Solid Edge part; units mm, degrees
sketch "Sketch1" plane through (0, 0, 0) normal (0, -1, 0) x (1, 0, 0)
  line L0 (0, 50.8) -> (0, 0)
  line L1 (0, 0) -> (50.8, 0)
  line L2 (50.8, 0) -> (50.8, 1.905)
  arc A0 (50.8, 1.905) -> (47.9425, 4.7625) centre (47.9425, 1.905) ccw
  line L3 (47.9425, 4.7625) -> (10.4775, 4.7625)
  arc A1 (10.4775, 4.7625) -> (4.7625, 10.4775) centre (10.4775, 10.4775) cw
  line L4 (4.7625, 10.4775) -> (4.7625, 47.9425)
  arc A2 (4.7625, 47.9425) -> (1.905, 50.8) centre (1.905, 47.9425) ccw
  line L5 (1.905, 50.8) -> (0, 50.8)
extrude "Protrusion1" add sketch "Sketch1" against normal blind 34.925
The listing builds one solid part. Answer for the finished solid, in the listing's coordinates (mm). A direction names the side the tool comes from. Coordinates: 2 decimals unless noted, no trailing zeros. Order: outer loops, then holes, each group sorted by start corner. A loop starts at its lowest first (then second) coordinate and runs counter-clockwise, first axis right, second up. Notation, with made-up numbers: (62, 26.25) -> (98, 26.25) arc R10 ccw to (98, 39.25) -> close; hole circle Ø2 at (29, 10). An arc over 180 degrees is marked (long way). Answer in a Markdown table with one row per item. Add a question column.
Item 1: Find section C-C (x = 27.5). Write down the section's boundary in (y, z) (1 decimal), then the cut area to 3 significant figures.
Item 2: Find section B-B (z = 11.5). Write down the section's boundary in (x, y) (1 decimal), then the cut area to 3 significant figures.
Item 3: Find the intervals of material crossed by L1, parallel to X at y = 6.5, z = 25; L2, parallel to X at y = 23.5, z = 7, in increasing order. Write a range as from..to.
Item 4: Each of these flat-tipped pins is pushed along its axis until it touches: P1, Ø8, axis at y = 10.5, z = 14, coming from the +X side; P2, Ø4, axis at x = 17.5, y = 22.5, coming from the +Z side. Where does it stop, or does it pass through?
Item 5: Find section A-A (y = 9.5). Write down the section's boundary in (x, z) (1 decimal), then the cut area to 3 significant figures.
Item 6: Which of the six approach directions +Z, -Z, +X, -X, +Y, -Y give full straight-line access (tool end or side, diameter ignored) to faces 1 (the face through (25, 17, 0)), 2 (the face through (29, 17, 4.762))?
Result set:
| question | item | result |
|---|---|---|
| 1 | outline | (0, 0) -> (34.9, 0) -> (34.9, 4.8) -> (0, 4.8) -> close |
| 1 | area | 166 mm² |
| 2 | outline | (0, 0) -> (4.8, 0) -> (4.8, 34.9) -> (0, 34.9) -> close |
| 2 | area | 166 mm² |
| 3 | L1 | x = 0..4.76 |
| 3 | L2 | x = 0..5.94 |
| 4 | P1 | stops at x = 4.78 |
| 4 | P2 | stops at z = 4.76 |
| 5 | outline | (0, 0) -> (50.8, 0) -> (50.8, 1.9) arc R2.9 ccw to (47.9, 4.8) -> (10.5, 4.8) arc R5.7 cw to (4.8, 10.5) -> (4.8, 47.9) arc R2.9 ccw to (1.9, 50.8) -> (0, 50.8) -> close |
| 5 | area | 465 mm² |
| 6 | face 1 | -Z, +X, -X, +Y, -Y |
| 6 | face 2 | +Z, +X, +Y, -Y |
